```python
from build123d import *

# Parameters (mm, degrees)
EXTRUDE_1_DEPTH             = 90
SKETCH_2_W                  = 90
SKETCH_2_H                  = 17.75
EXTRUDE_2_DEPTH             = 8.2
SKETCH_3_W                  = 90
SKETCH_3_H                  = 102.45
EXTRUDE_3_DEPTH             = 8.2
SKETCH_4_W                  = 3.95
SKETCH_4_H                  = 2.25
CUT_EXTRUDE_1_DEPTH         = 171.45954982
SKETCH_5_W                  = 3.95
SKETCH_5_H                  = 29.5
CUT_EXTRUDE_2_DEPTH         = 171.45954982
SKETCH_6_W                  = 3.95
SKETCH_6_H                  = 9
CUT_EXTRUDE_3_DEPTH         = 171.45954982
SKETCH_7_W                  = 3.95
SKETCH_7_H                  = 29.5
CUT_EXTRUDE_4_DEPTH         = 171.45954982
SKETCH_8_W                  = 3.95
SKETCH_8_H                  = 6.2
CUT_EXTRUDE_5_DEPTH         = 171.45954982
SKETCH_9_W                  = 2.25
SKETCH_9_H                  = 3.95
CUT_EXTRUDE_6_DEPTH         = 171.45954982
SKETCH_10_W                 = 4.5
SKETCH_10_H                 = 3.95
CUT_EXTRUDE_7_DEPTH         = 171.45954982
SKETCH_11_W                 = 2.25
SKETCH_11_H                 = 3.95
CUT_EXTRUDE_8_DEPTH         = 171.45954982
SKETCH_12_W                 = 20.2
SKETCH_12_H                 = 96.7
CUT_EXTRUDE_9_DEPTH         = 86
HOLE_WIZARD_8_3_8_3_1_D     = 8.3
HOLE_WIZARD_8_3_8_3_1_DEPTH = 3.2
HOLE_WIZARD_4_5_4_5_1_D     = 4.5
HOLE_WIZARD_2_5_2_5_1_D     = 2.5
SKETCH_19_R                 = 4.5030807
EXTRUDE_4_DEPTH             = 3
SKETCH_20_R                 = 1.649948342
SKETCH_20_R_2               = 1.660581376
SKETCH_20_R_3               = 1.430745594
SKETCH_20_R_4               = 1.573250385
SKETCH_20_R_5               = 1.502029841
SKETCH_20_R_6               = 1.53795619
EXTRUDE_5_DEPTH             = 90
CUT_EXTRUDE_10_DEPTH        = 112
CUT_EXTRUDE_10_DEPTH_BACK   = 112
EXTRUDE_6_DEPTH             = 20
EXTRUDE_6_DEPTH_BACK        = 3
SKETCH_22_W                 = 10.1
SKETCH_22_H                 = 96.7
SKETCH_23_W                 = 66
SKETCH_23_H                 = 10.1
EXTRUDE_7_DEPTH             = 10
SKETCH_24_W                 = 66
SKETCH_24_H                 = 10.1
EXTRUDE_8_DEPTH             = 10
SKETCH_25_W                 = 10.1
SKETCH_25_H                 = 76.7
EXTRUDE_9_DEPTH             = 20
SKETCH_26_W                 = 11
SKETCH_26_H                 = 98.5
EXTRUDE_10_DEPTH            = 25
CUT_EXTRUDE_13_DEPTH        = 123
EXTRUDE_11_DEPTH            = 78
EXTRUDE_11_DEPTH_BACK       = 2
SKETCH_29_W                 = 46
SKETCH_29_H                 = 10.1


with BuildPart() as part:
    # Эскиз1 → Бобышка-Вытянуть1 (new body)
    with BuildSketch(Plane(origin=(90, 0, 0), x_dir=(0, 0, -1), z_dir=(1, 0, 0))):
        with BuildLine():
            Line((6.75, 40.906238208), (6.75, 135.75))
            Line((6.75, 135.75), (-11.593761792, 135.75))
            ThreePointArc((-11.593761792, 135.75), (-15.325, 134.5), (-11.593761793, 133.25))
            Line((-11.593761793, 133.25), (-11, 133.25))
            Line((-11, 133.25), (-11, 99.75))
            Line((-11, 99.75), (-11.593761792, 99.75))
            ThreePointArc((-11.593761792, 99.75), (-15.325, 98.5), (-11.593761792, 97.25))
            Line((-11.593761792, 97.25), (-11, 97.25))
            Line((-11, 97.25), (-11, 84.25))
            Line((-11, 84.25), (-11.593761792, 84.25))
            ThreePointArc((-11.593761792, 84.25), (-15.325, 83), (-11.593761792, 81.75))
            Line((-11.593761792, 81.75), (-11, 81.75))
            Line((-11, 81.75), (-11, 48.25))
            Line((-11, 48.25), (-11.593761792, 48.25))
            ThreePointArc((-11.593761792, 48.25), (-15.325, 47), (-11.593761792, 45.75))
            Line((-11.593761792, 45.75), (-11, 45.75))
            Line((-11, 45.75), (-11, 41.5))
            Line((-11, 41.5), (-6.75, 41.5))
            Line((-6.75, 41.5), (-6.75, 40.906238208))
            ThreePointArc((-6.75, 40.906238208), (-5.5, 37.175), (-4.25, 40.906238208))
            Line((-4.25, 40.906238208), (-4.25, 41.5))
            Line((-4.25, 41.5), (4.25, 41.5))
            Line((4.25, 41.5), (4.25, 40.906238208))
            ThreePointArc((4.25, 40.906238208), (5.5, 37.175), (6.75, 40.906238208))
        make_face()
    extrude(amount=-EXTRUDE_1_DEPTH)

    # Эскиз2 → Бобышка-Вытянуть2 (add)
    with BuildSketch(Plane(origin=(0, 135.75, 0), x_dir=(-1, 0, 0), z_dir=(0, 1, 0))):
        with Locations((-45, 2.125)):
            Rectangle(SKETCH_2_W, SKETCH_2_H)
    extrude(amount=EXTRUDE_2_DEPTH)

    # Эскиз3 → Бобышка-Вытянуть3 (add)
    with BuildSketch(Plane(origin=(0, 0, -6.75), x_dir=(-1, 0, 0), z_dir=(0, 0, -1))):
        with Locations((-45, 92.725)):
            Rectangle(SKETCH_3_W, SKETCH_3_H)
    extrude(amount=EXTRUDE_3_DEPTH)

    # Эскиз4 → Вырез-Вытянуть1 (cut, through all)
    with BuildSketch(Plane.ZY):
        with Locations((-12.975, 42.625)):
            Rectangle(SKETCH_4_W, SKETCH_4_H)
    extrude(amount=-CUT_EXTRUDE_1_DEPTH, mode=Mode.SUBTRACT)

    # Эскиз5 → Вырез-Вытянуть2 (cut, through all)
    with BuildSketch(Plane.ZY):
        with Locations((-12.975, 65)):
            Rectangle(SKETCH_5_W, SKETCH_5_H)
    extrude(amount=-CUT_EXTRUDE_2_DEPTH, mode=Mode.SUBTRACT)

    # Эскиз6 → Вырез-Вытянуть3 (cut, through all)
    with BuildSketch(Plane.ZY):
        with Locations((-12.975, 90.75)):
            Rectangle(SKETCH_6_W, SKETCH_6_H)
    extrude(amount=-CUT_EXTRUDE_3_DEPTH, mode=Mode.SUBTRACT)

    # Эскиз7 → Вырез-Вытянуть4 (cut, through all)
    with BuildSketch(Plane.ZY):
        with Locations((-12.975, 116.5)):
            Rectangle(SKETCH_7_W, SKETCH_7_H)
    extrude(amount=-CUT_EXTRUDE_4_DEPTH, mode=Mode.SUBTRACT)

    # Эскиз8 → Вырез-Вытянуть5 (cut, through all)
    with BuildSketch(Plane.ZY):
        with Locations((-12.975, 140.85)):
            Rectangle(SKETCH_8_W, SKETCH_8_H)
    extrude(amount=-CUT_EXTRUDE_5_DEPTH, mode=Mode.SUBTRACT)

    # Эскиз9 → Вырез-Вытянуть6 (cut, through all)
    with BuildSketch(Plane.ZY):
        with Locations((-9.875, 141.975)):
            Rectangle(SKETCH_9_W, SKETCH_9_H)
    extrude(amount=-CUT_EXTRUDE_6_DEPTH, mode=Mode.SUBTRACT)

    # Эскиз10 → Вырез-Вытянуть7 (cut, through all)
    with BuildSketch(Plane.ZY):
        with Locations((0, 141.975)):
            Rectangle(SKETCH_10_W, SKETCH_10_H)
    extrude(amount=-CUT_EXTRUDE_7_DEPTH, mode=Mode.SUBTRACT)

    # Эскиз11 → Вырез-Вытянуть8 (cut, through all)
    with BuildSketch(Plane.ZY):
        with Locations((9.875, 141.975)):
            Rectangle(SKETCH_11_W, SKETCH_11_H)
    extrude(amount=-CUT_EXTRUDE_8_DEPTH, mode=Mode.SUBTRACT)

    # Эскиз12 → Вырез-Вытянуть9 (cut)
    with BuildSketch(Plane(origin=(90, 0, 0), x_dir=(0, 0, -1), z_dir=(1, 0, 0))):
        with Locations((0, 90.75)):
            Rectangle(SKETCH_12_W, SKETCH_12_H)
    extrude(amount=-CUT_EXTRUDE_9_DEPTH, mode=Mode.SUBTRACT)

    # Диаметр отверстия Ø8.3 (8.3)1
    with Locations(Plane.ZY):
        with Locations((0, 90)):
            Hole(HOLE_WIZARD_8_3_8_3_1_D / 2, depth=HOLE_WIZARD_8_3_8_3_1_DEPTH)

    # Диаметр отверстия Ø4.5 (4.5)1 (through all)
    with Locations(Plane.ZY):
        with Locations((-13.25, 47), (-13.25, 83), (-13.25, 98.5), (-13.25, 134.5), (-5.5, 142.25), (5.5, 142.25)):
            Hole(HOLE_WIZARD_4_5_4_5_1_D / 2)

    # Диаметр отверстия Ø2.5 (2.5)1 (through all)
    with Locations(Plane(origin=(90, 0, 0), x_dir=(0, 0, -1), z_dir=(1, 0, 0))):
        with Locations((-13.25, 98.5), (-13.25, 134.5), (-13.25, 47), (-13.25, 83), (5.5, 39.25), (-5.5, 39.25)):
            Hole(HOLE_WIZARD_2_5_2_5_1_D / 2)

    # Эскиз19 → Бобышка-Вытянуть4 (add)
    with BuildSketch(Plane.ZY):
        with Locations((0, 90)):
            Circle(SKETCH_19_R)
    extrude(amount=-EXTRUDE_4_DEPTH)

    # Эскиз20 → Бобышка-Вытянуть5 (add)
    with BuildSketch(Plane(origin=(90, 0, 0), x_dir=(0, 0, -1), z_dir=(1, 0, 0))):
        with Locations((-13.25, 134.5)):
            Circle(SKETCH_20_R)
        with Locations((-13.25, 98.5)):
            Circle(SKETCH_20_R_2)
        with Locations((-13.25, 83)):
            Circle(SKETCH_20_R_3)
        with Locations((-13.25, 47)):
            Circle(SKETCH_20_R_4)
        with Locations((-5.5, 39.25)):
            Circle(SKETCH_20_R_5)
        with Locations((5.5, 39.25)):
            Circle(SKETCH_20_R_6)
    extrude(amount=-EXTRUDE_5_DEPTH)

    # Эскиз21 → Вырез-Вытянуть10 (cut, two sides: drawn at the far end of the back side and taken through both)
    with BuildSketch(Plane(origin=(4, 0, 0), x_dir=(0, 0, -1), z_dir=(1, 0, 0)).offset(-CUT_EXTRUDE_10_DEPTH_BACK)):
        Polygon((0, 140), (0, 41.5), (0, 35.614345614), (18.747428666, 35.614345614), (18.747428666, 145.957941917), (0, 145.957941917), align=None)
    extrude(amount=CUT_EXTRUDE_10_DEPTH + CUT_EXTRUDE_10_DEPTH_BACK, mode=Mode.SUBTRACT)

    # Эскиз22 → Бобышка-Вытянуть6 (add, two sides: drawn at the far end of the back side and taken through both)
    with BuildSketch(Plane(origin=(4, 0, 0), x_dir=(0, 0, -1), z_dir=(1, 0, 0)).offset(-EXTRUDE_6_DEPTH_BACK)):
        with Locations((-5.05, 90.75)):
            Rectangle(SKETCH_22_W, SKETCH_22_H)
    extrude(amount=EXTRUDE_6_DEPTH + EXTRUDE_6_DEPTH_BACK)

    # Эскиз23 → Бобышка-Вытянуть7 (add)
    with BuildSketch(Plane.XZ.offset(-139.1)):
        with Locations((57, 5.05)):
            Rectangle(SKETCH_23_W, SKETCH_23_H)
    extrude(amount=EXTRUDE_7_DEPTH)

    # Эскиз24 → Бобышка-Вытянуть8 (add)
    with BuildSketch(Plane(origin=(0, 42.4, 0), x_dir=(1, 0, 0), z_dir=(0, 1, 0))):
        with Locations((57, -5.05)):
            Rectangle(SKETCH_24_W, SKETCH_24_H)
    extrude(amount=EXTRUDE_8_DEPTH)

    # Эскиз25 → Бобышка-Вытянуть9 (add)
    with BuildSketch(Plane(origin=(90, 0, 0), x_dir=(0, 0, -1), z_dir=(1, 0, 0))):
        with Locations((-5.05, 90.75)):
            Rectangle(SKETCH_25_W, SKETCH_25_H)
    extrude(amount=-EXTRUDE_9_DEPTH)

    # Эскиз26 → Бобышка-Вытянуть10 (add)
    with BuildSketch(Plane(origin=(90, 0, 0), x_dir=(0, 0, -1), z_dir=(1, 0, 0))):
        with Locations((-5.5, 90.75)):
            Rectangle(SKETCH_26_W, SKETCH_26_H)
    extrude(amount=EXTRUDE_10_DEPTH)

    # Эскиз27 → Вырез-Вытянуть13 (cut)
    with BuildSketch(Plane.XZ.offset(-41.5)):
        Polygon((90, 11), (115, 0), (115, 11), align=None)
    extrude(amount=-CUT_EXTRUDE_13_DEPTH, mode=Mode.SUBTRACT)

    # Эскиз29 → Бобышка-Вытянуть11 (add, two sides: drawn at the far end of the back side and taken through both)
    with BuildSketch(Plane.XZ.offset(-129.1).offset(-EXTRUDE_11_DEPTH_BACK)):
        with Locations((47, 5.05)):
            Rectangle(SKETCH_29_W, SKETCH_29_H)
    extrude(amount=EXTRUDE_11_DEPTH + EXTRUDE_11_DEPTH_BACK)


solid = part.part
```
Geometry check sheet. Reference: the model listing, model coordinates, mm. A direction names the side the tool comes from. Coordinates: 2 decimals unless noted, no trailing zeros. Order: outer loops, then holes, each group sorted by start corner. A loop starts at its lowest first (then second) coordinate and runs counter-clockwise, first axis right, second up. Notation, with made-up numbers: (-19.75, -1) - (15.25, -1) arc R15 cw to (15.25, 28) - close; hole circle Ø3 at (0, 82.5). An arc over 180 degrees is marked (long way). Answer in a Markdown table with one row per item. Add a question column.
1. Section check A-A (y = 142.25). Enter the section's corners in (x, z), plus the area to 3 significant figures.
2. Gauge pin test, flat ends, axial feed: pin 1 Ø1 at (y, z) = (91, 3) entering from -X; pin 2 Ø2 at (y, z) = (133.5, 13) entering from +X; pin 3 Ø3 at (x, y) = (67, 142) entering from -Z; pin 4 Ø4 at (x, y) = (50, 94) entering from +Z. Record the tip position at first contact, or that the pin passes through.
3. Section check D-D (y = 68). Enter the section's corners in (x, z), plus the area to 3 significant figures.
4. Access from +Z, -Z, +X, -X, +Y, -Y to the whole of each face (thin tool, end or side, straight path). Record for faces 3 (the face through (90, 142, 3)), 4 (the face through (44, 44, 11)), 5 (the face through (90, 39, 6)), 6 (the face through (44, 142, 2.25)).
5. Section check C-C (y = 39.25). Enter the section's corners in (x, z) (3 decimals).
6. Draft check along Y on faces 1 (the face through (90, 83, 13)), 2 (the face through (44, 116, 11)). Enter one of: +Y half, -Y half, draft (parallel to the pull), parting line (faces both ways), or undercut.
7. Material ranges on L1, parallel to Y at x = 63, z = 11.5; L2, parallel to Z at x = 55, y = 142; L3, parallel to Y at x = 7.5, z = 14, recorded low to high. Write a range as [from, to].
Data:
| question | item | result |
|---|---|---|
| 1 | outline | (0, 2.25) - (90, 2.25) - (90, 3.25) - (0, 3.25) - close; (0, 7.75) - (90, 7.75) - (90, 8.75) - (0, 8.75) - close |
| 1 | area | 180 mm² |
| 2 | pin 1 | stops at x = 0 |
| 2 | pin 2 | stops at x = 90 |
| 2 | pin 3 | stops at z = 2.25 |
| 2 | pin 4 | stops at z = 11 |
| 3 | outline | (0, 0) - (115, 0) - (90, 11) - (0, 11) - close |
| 3 | area | 1,130 mm² |
| 4 | face 3 | +Z, -Z, +X, +Y |
| 4 | face 4 | +X, -X, -Y |
| 4 | face 5 | +Z, -Z, +X, -Y |
| 4 | face 6 | -Z, +X, -X, +Y |
| 5 | outline | (0, 3.425) - (90, 3.425) - (90, 7.575) - (0, 7.575) - close |
| 6 | face 1 | draft |
| 6 | face 2 | undercut |
| 7 | L1 | y = [45.75, 48.25], [81.75, 84.25], [97.25, 99.75], [133.25, 135.75] |
| 7 | L2 | z = [2.25, 3.26], [7.74, 8.75] |
| 7 | L3 | y = [45.07, 48.93], [81.07, 84.93], [96.57, 100.43], [132.57, 136.43] |
